from build123d import *

# Parameters (mm, degrees)
ESQUISSE1_R        = 2.15
BOSS_EXTRU_1_DEPTH = 165


with BuildPart() as part:
    # Esquisse1 → Boss.-Extru.1 (new body)
    with BuildSketch(Plane(origin=(0, 0, 0), x_dir=(-1, 0, 0), z_dir=(0, 0, -1))):
        with BuildLine():
            Line((-12.499999997, 0.800000003), (-12.499999998, 1.500000003))
            ThreePointArc((-12.499999998, 1.500000003), (-12.587867964, 1.712132039), (-12.8, 1.800000005))
            Line((-12.8, 1.800000005), (-14.9175884, 1.800000005))
            ThreePointArc((-14.9175884, 1.800000005), (-15.686636444, 2.31386148), (-15.50619229, 3.2210155))
            Line((-15.50619229, 3.2210155), (-13.25588745, 5.47132034))
            ThreePointArc((-13.25588745, 5.47132034), (-12.282617404, 6.121638593), (-11.134567108, 6.349999996))
            Line((-11.134567108, 6.349999996), (-8.865432907, 6.349999996))
            ThreePointArc((-8.865432907, 6.349999996), (-7.717382611, 6.121638594), (-6.744112567, 5.471320341))
            Line((-6.744112567, 5.471320341), (-4.493807729, 3.221015503))
            ThreePointArc((-4.493807729, 3.221015503), (-4.313363575, 2.313861481), (-5.082411621, 1.800000005))
            Line((-5.082411621, 1.800000005), (-7.20000001, 1.800000005))
            ThreePointArc((-7.20000001, 1.800000005), (-7.412132045, 1.71213204), (-7.50000001, 1.500000005))
            Line((-7.50000001, 1.500000005), (-7.50000001, 0.8))
            ThreePointArc((-7.50000001, 0.8), (-7.265685435, 0.234314575), (-6.70000001, 0))
            Line((-6.70000001, 0), (-2, 0))
            ThreePointArc((-2, 0), (-0.585786438, 0.585786438), (0, 2))
            Line((0, 2), (0, 6.699999998))
            ThreePointArc((0, 6.699999998), (-0.234314576, 7.265685424), (-0.800000003, 7.5))
            Line((-0.800000003, 7.5), (-1.50000001, 7.5))
            ThreePointArc((-1.50000001, 7.5), (-1.712132046, 7.412132033), (-1.800000013, 7.199999997))
            Line((-1.800000013, 7.199999997), (-1.800000013, 5.082411603))
            ThreePointArc((-1.800000013, 5.082411603), (-2.313861487, 4.31336356), (-3.221015507, 4.493807713))
            Line((-3.221015507, 4.493807713), (-5.471320347, 6.744112553))
            ThreePointArc((-5.471320347, 6.744112553), (-6.1216386, 7.717382599), (-6.350000003, 8.865432896))
            Line((-6.350000003, 8.865432896), (-6.350000003, 11.134567102))
            ThreePointArc((-6.350000003, 11.134567102), (-6.121638601, 12.282617397), (-5.471320348, 13.255887442))
            Line((-5.471320348, 13.255887442), (-3.221015512, 15.506192278))
            ThreePointArc((-3.221015512, 15.506192278), (-2.313861489, 15.686636432), (-1.800000013, 14.917588386))
            Line((-1.800000013, 14.917588386), (-1.800000013, 12.799999998))
            ThreePointArc((-1.800000013, 12.799999998), (-1.712132047, 12.587867963), (-1.500000013, 12.499999997))
            Line((-1.500000013, 12.499999997), (-0.8, 12.499999997))
            ThreePointArc((-0.8, 12.499999997), (-0.234314575, 12.734314573), (0, 13.299999998))
            Line((0, 13.299999998), (0, 18))
            ThreePointArc((0, 18), (-0.585786438, 19.414213562), (-2, 20))
            Line((-2, 20), (-6.700000008, 20))
            ThreePointArc((-6.700000008, 20), (-7.265685435, 19.765685424), (-7.50000001, 19.199999998))
            Line((-7.50000001, 19.199999998), (-7.50000001, 18.500000005))
            ThreePointArc((-7.50000001, 18.500000005), (-7.412132044, 18.287867969), (-7.200000008, 18.200000003))
            Line((-7.200000008, 18.200000003), (-5.082411594, 18.200000003))
            ThreePointArc((-5.082411594, 18.200000003), (-4.313363546, 17.686138526), (-4.493807701, 16.778984501))
            Line((-4.493807701, 16.778984501), (-6.744112542, 14.528679659))
            ThreePointArc((-6.744112542, 14.528679659), (-7.717382588, 13.878361406), (-8.865432885, 13.650000003))
            Line((-8.865432885, 13.650000003), (-11.134567112, 13.650000003))
            ThreePointArc((-11.134567112, 13.650000003), (-12.282617407, 13.878361405), (-13.255887452, 14.528679658))
            Line((-13.255887452, 14.528679658), (-15.506192292, 16.778984498))
            ThreePointArc((-15.506192292, 16.778984498), (-15.686636447, 17.686138525), (-14.917588397, 18.200000002))
            Line((-14.917588397, 18.200000002), (-12.799999998, 18.200000003))
            ThreePointArc((-12.799999998, 18.200000003), (-12.587867963, 18.287867968), (-12.499999997, 18.500000002))
            Line((-12.499999997, 18.500000002), (-12.499999997, 19.2))
            ThreePointArc((-12.499999997, 19.2), (-12.734314573, 19.765685425), (-13.299999998, 20))
            Line((-13.299999998, 20), (-18, 20))
            ThreePointArc((-18, 20), (-19.414213562, 19.414213562), (-20, 18))
            Line((-20, 18), (-20, 13.3))
            ThreePointArc((-20, 13.3), (-19.765685424, 12.734314573), (-19.199999998, 12.499999997))
            Line((-19.199999998, 12.499999997), (-18.500000003, 12.499999997))
            ThreePointArc((-18.500000003, 12.499999997), (-18.287867967, 12.587867964), (-18.2, 12.8))
            Line((-18.2, 12.8), (-18.2, 14.91758839))
            ThreePointArc((-18.2, 14.91758839), (-17.686138526, 15.686636434), (-16.778984506, 15.50619228))
            Line((-16.778984506, 15.50619228), (-14.528679657, 13.255887431))
            ThreePointArc((-14.528679657, 13.255887431), (-13.878361403, 12.282617385), (-13.650000001, 11.134567088))
            Line((-13.650000001, 11.134567088), (-13.650000001, 8.865432886))
            ThreePointArc((-13.650000001, 8.865432886), (-13.878361403, 7.717382591), (-14.528679656, 6.744112546))
            Line((-14.528679656, 6.744112546), (-16.778984496, 4.493807706))
            ThreePointArc((-16.778984496, 4.493807706), (-17.686138522, 4.313363551), (-18.2, 5.0824116))
            Line((-18.2, 5.0824116), (-18.2, 7.2))
            ThreePointArc((-18.2, 7.2), (-18.287867966, 7.412132034), (-18.5, 7.5))
            Line((-18.5, 7.5), (-19.2, 7.5))
            ThreePointArc((-19.2, 7.5), (-19.765685425, 7.265685425), (-20, 6.7))
            Line((-20, 6.7), (-20, 2))
            ThreePointArc((-20, 2), (-19.414213562, 0.585786438), (-18, 0))
            Line((-18, 0), (-13.3, 0))
            ThreePointArc((-13.3, 0), (-12.734314573, 0.234314576), (-12.499999997, 0.800000003))
        make_face()
        with Locations(Location((-10, 10, 0), (0, 0, 180))):
            Circle(ESQUISSE1_R, mode=Mode.SUBTRACT)
    extrude(amount=-BOSS_EXTRU_1_DEPTH)


solid = part.part
The listing builds one solid part. Answer for the finished solid, in the listing's coordinates (mm). Give positions to 0.01 mm unless a question says otherwise; leave off trailing zeros.
1) For a pull along Y with two mould halves and no side action, classify faces 1 (the face through (20, 4, 81)), 2 (the face through (9.72, 7.87, 81.34)), 3 (the face through (4, 0, 81)) as pulls with the +Y half, pulls with the -Y half, needs draft (parallel to the pull), parting line crosses it, or undercut.
2) Find the intervals of material crossed by L1, parallel to Y at x = 10, z = 120; L2, parallel to X at y = 4.75, z = 23, in increasing order.
3) Given P1, Ø0.8, axis at x = 1, z = 111.5, coming from the -Y side; P2, Ø1.1, axis at y = 9.5, z = 62.5, coming from the +X side; P3, Ø2.5, axis at x = 10.5, z = 60.5, coming from the +Y side, each flat-ended and moving along its own axis, determine where each tip first touches the part or whether it passes through.
Response:
1. face 1: needs draft
1. face 2: undercut
1. face 3: pulls with the -Y half
2. L1: y = 6.35 to 7.85, 12.15 to 13.65
2. L2: x = 0 to 1.87, 3.48 to 6.02, 13.98 to 16.52, 18.13 to 20
3. P1: stops at y = 0.09
3. P2: stops at x = 13.65
3. P3: stops at y = 13.71
